Input: part model. Units: mm. Frame: model coordinates. Give positions to 0.01 mm unless a question says otherwise; leave off trailing zeros. Loops run counter-clockwise (first coordinate to the right, second up) from the corner with the lowest first, then second, coordinate; pieces in that order, holes last. Notation, with made-up numbers: (-7, 57.25) - (31, 57.25) arc R22 cw to (31, 70.25) - close; hole circle Ø1 at (37, -11.5). An arc over 180 degrees is marked (long way). Answer as a JSON object with one key per item and string values. Group by question number.
(1) Section query D-D (z = 15). Return loops of the section in (x, y), plus the area to 3 significant figures.
(2) Section query B-B (y = 22). Return loops of the section in (x, z), plus the area to 3 significant figures.
(3) Material intervals for L1, parallel to Z at x = 93.5, y = 7; L2, parallel to Y at x = 55, z = 5.5; L3, parallel to X at y = 15, z = 4, sorted ascending.
(4) Section query A-A (x = 63.7). Return loops of the section in (y, z).
(5) Section query C-C (x = 44). Return loops of the section in (y, z), plus the area to 3 significant figures.
(6) Pin query (flat end, axial travel): P1, Ø1, axis at y = 25.5, z = 22.5, coming from the -X side; P2, Ø1.5, axis at y = 8, z = 19, coming from the -X side. Return the tip coordinate at first contact, or that it passes through.
Autodesk Inventor part; units mm, degrees
ref_plane "YZ Plane" through (0, 0, 0) normal (1, 0, 0) x (0, 1, 0)
ref_plane "XZ Plane" through (0, 0, 0) normal (0, 1, 0) x (-1, 0, 0)
ref_plane "XY Plane" through (0, 0, 0) normal (0, 0, 1) x (1, 0, 0)
sketch "Sketch1" plane through (0, 0, 0) normal (0, 0, 1) x (1, 0, 0)
  line L0 (0, 2) -> (100, 2) construction
  line L1 (0, 2) -> (0, 18) construction
  line L2 (12, 18) -> (0, 18) construction
  arc A0 (12, 18) -> (28, 18) centre (20, 18) ccw construction
  line L3 (38, 18) -> (28, 18) construction
  arc A1 (38, 18) -> (62, 18) centre (50, 18) ccw construction
  line L4 (72, 18) -> (62, 18) construction
  arc A2 (72, 18) -> (88, 18) centre (80, 18) ccw construction
  line L5 (100, 18) -> (88, 18) construction
  line L6 (100, 2) -> (100, 18) construction
  line L7 (100, 34) -> (0, 34) construction
  line L8 (100, 34) -> (100, 18) construction
  line L9 (88, 18) -> (100, 18) construction
  arc A3 (88, 18) -> (72, 18) centre (80, 18) ccw construction
  line L10 (62, 18) -> (72, 18) construction
  arc A4 (62, 18) -> (38, 18) centre (50, 18) ccw construction
  line L11 (28, 18) -> (38, 18) construction
  arc A5 (28, 18) -> (12, 18) centre (20, 18) ccw construction
  line L12 (0, 18) -> (12, 18) construction
  line L13 (0, 34) -> (0, 18) construction
  line L14 (100, 2) -> (100, 0) construction
  line L15 (100, 0) -> (0, 0) construction
  line L16 (0, 0) -> (0, 2) construction
  line L17 (0, 2) -> (100, 2) construction
  line L18 (0, 34) -> (0, 36) construction
  line L19 (0, 36) -> (100, 36) construction
  line L20 (100, 36) -> (100, 34) construction
  line L21 (100, 34) -> (0, 34) construction
  line L22 (100, 36) -> (100, 0)
  line L23 (100, 0) -> (55, 0)
  line L24 (19, 36) -> (100, 36)
  circle A6 centre (80, 18) radius 8
  line L25 (72.0156, 18.5) -> (36.5, 18.5)
  line L26 (37.5, 17.5) -> (72.0156, 17.5)
  line L27 (55, 0) -> (37.5, 17.5)
  line L28 (36.5, 18.5) -> (19, 36)
  line L29 (55.9956, 18.5) -> (55.9956, 17.5) construction
  line L30 (36.5, 18.5) -> (37.5, 17.5) construction
  point P0 (55.9956, 18)
  dimension "d1" = 45
  dimension "d3" = 1
  dimension "d4" = 45
extrude "Extrusion1" add sketch "Sketch1" along normal blind 32 contours L22 L23 L27 L26 A6 L25 L28 L24
sketch "Sketch2" plane through (55, 0, 0) normal (0, -1, 0) x (1, 0, 0)
  circle A0 centre (38.5, 25.5) radius 3
  circle A1 centre (38.5, 6.5) radius 3
  circle A2 centre (8.7, 16) radius 3
  point P0 (-55, 0)
extrude "Extrusion2" cut sketch "Sketch2" against normal through all
chamfer "Chamfer1" distance 2 angle 45 4 edges at (77.5, 0, 0) (59.5, 36, 0) (77.5, 0, 32) (59.5, 36, 32)
properties part number "AXTTS" material "PC/ABS Plastic"
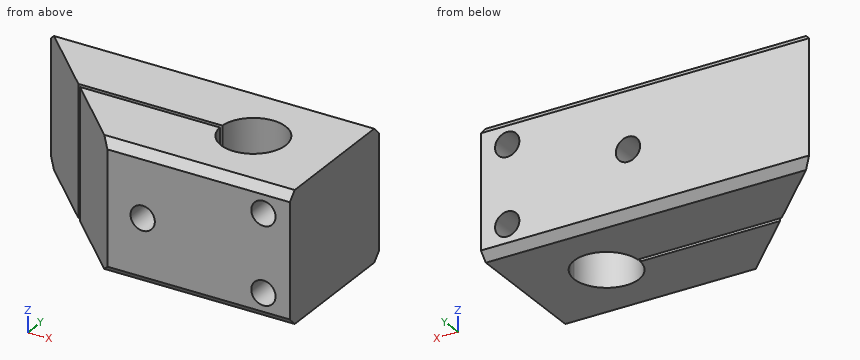
Recorded:
{
 "1": {"outline": "(19, 36) - (36.5, 18.5) - (60.87, 18.5) - (60.87, 36) - close; (37.5, 17.5) - (55, 0) - (60.87, 0) - (60.87, 17.5) - close; (66.53, 0) - (100, 0) - (100, 36) - (66.53, 36) - (66.53, 18.5) - (72.02, 18.5) arc R8 cw (long way) to (72.02, 17.5) - (66.53, 17.5) - close", "area": "1,830 mm^2"},
 "2": {"outline": "(33, 0) - (73.07, 0) - (73.07, 32) - (33, 32) - close; (86.93, 0) - (100, 0) - (100, 32) - (86.93, 32) - close; hole circle Ø6 at (63.7, 16); hole circle Ø6 at (93.5, 6.5); hole circle Ø6 at (93.5, 25.5)", "area": "1,620 mm^2"},
 "3": {"L1": "z = 0 to 3.5, 9.5 to 22.5, 28.5 to 32", "L2": "y = 0 to 17.5, 18.5 to 36", "L3": "x = 40 to 72.58, 87.42 to 91.84, 95.16 to 100"},
 "4": {"outline": "(0, 2) - (2, 0) - (17.5, 0) - (17.5, 13) - (0, 13) - close; (0, 19) - (17.5, 19) - (17.5, 32) - (2, 32) - (0, 30) - close; (18.5, 0) - (34, 0) - (36, 2) - (36, 13) - (18.5, 13) - close; (18.5, 19) - (36, 19) - (36, 30) - (34, 32) - (18.5, 32) - close"},
 "5": {"outline": "(11, 0) - (17.5, 0) - (17.5, 32) - (11, 32) - close; (18.5, 0) - (34, 0) - (36, 2) - (36, 30) - (34, 32) - (18.5, 32) - close", "area": "764 mm^2"},
 "6": {"P1": "stops at x = 29", "P2": "stops at x = 46.25"}
}
